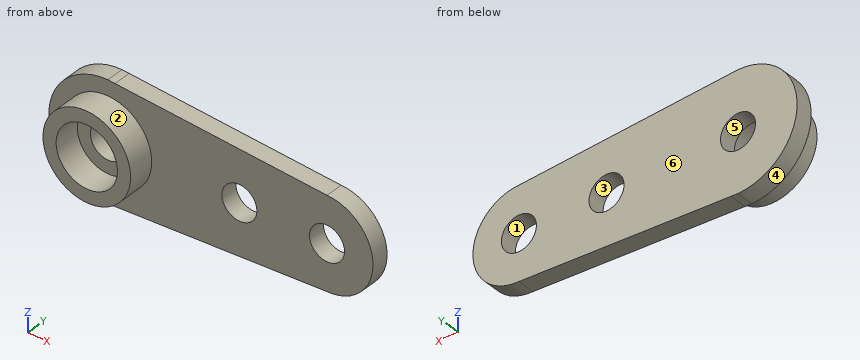
```python
from build123d import *

# Parameters (mm, degrees)
SKETCH_2_R      = 1
EXTRUDE_1_DEPTH = 1
SKETCH_3_R      = 2.5
SKETCH_3_R_2    = 1.75
EXTRUDE_2_DEPTH = 1.5


with BuildPart() as part:
    # 草图2 → 凸台-拉伸1 (new body)
    with BuildSketch(Plane(origin=(0, 0, 0), x_dir=(1, 0, 0), z_dir=(0, 1, 0))):
        with BuildLine():
            Line((0.40354723, 3.350787166), (0, 3.375))
            ThreePointArc((0, 3.375), (-3.375, 0), (0, -3.375))
            Line((0, -3.375), (0.40354723, -3.350787166))
            Line((0.40354723, -3.350787166), (12.5, -2.625))
            ThreePointArc((12.5, -2.625), (15.125, 0), (12.5, 2.625))
            Line((12.5, 2.625), (0.40354723, 3.350787166))
        make_face()
        with Locations(Location((0, 0, 0), (0, 0, 270))):
            Circle(SKETCH_2_R, mode=Mode.SUBTRACT)
        with Locations(Location((7.5, 0, 0), (0, 0, 270))):
            Circle(SKETCH_2_R, mode=Mode.SUBTRACT)
        with Locations(Location((12.5, 0, 0), (0, 0, 270))):
            Circle(SKETCH_2_R, mode=Mode.SUBTRACT)
    extrude(amount=EXTRUDE_1_DEPTH)

    # 草图3 → 凸台-拉伸2 (add)
    with BuildSketch(Plane(origin=(0, 0, 0), x_dir=(1, 0, 0), z_dir=(0, 1, 0))):
        with Locations(Location((0, 0, 0), (0, 0, 270))):
            Circle(SKETCH_3_R)
        with Locations(Location((0, 0, 0), (0, 0, 270))):
            Circle(SKETCH_3_R_2, mode=Mode.SUBTRACT)
    extrude(amount=-EXTRUDE_2_DEPTH)


solid = part.part
```
CAD build for the part. Positions are in the model's coordinates, mm. Face numbers are marked on the shaded views. A direction names the side the tool comes from. Coordinates: 2 decimals unless noted, no trailing zeros. Write each loop counter-clockwise with the first axis right and the second up, starting at its lowest first coordinate (ties: lowest second). Pieces come first, ordered by that corner, then holes.
(1) Drill centre lines: probe 1 along X at (y, z) = (0.7, 0) (3 decimals); probe 2 along Y at (x, z) = (10, 1.5); probe 3 along X at (y, z) = (-1.2, -1). Where is each one in solid material? Low to high.
(2) Flat gauge pin, fed straight in: pin 1 (4 mm diameter, centred on x = 5.5, z = -2, fed in from -Y). Where does the tip first touch, or does it go through?
(3) Cut at A-A, the plane z = 0. List the corners of the cut face in (x, y) (3 decimals).
(4) 3-axis set-ups, long thin cutter, end or side, ignore diameter. For the marked faces 1 and 2: which of +Z, -Z, +X, -X, +Y, -Y reach the whole face in a straight line?
(5) Cut at C-C, the plane x = 6.75. List the corners of the cut face in (y, z), and give its area (3 significant figures).
(6) Two-plate mould, pull along X, no slides. Class the marked faces 3, 4, 5 and 6: +X half, -X half, draft (parallel to the pull), parting line (faces both ways), or undercut.
(7) Cut at B-B, the plane y = 0.2. List the corners of the cut face in (x, z) (3 decimals).
(8) Cut at D-D, the plane x = 9.75. List the corners of the cut face in (y, z).
Geometry says:
1. probe 1: x = -3.375 to -1, 1 to 6.5, 8.5 to 11.5, 13.5 to 15.125
1. probe 2: y = 0 to 1
1. probe 3: x = -2.29 to -1.44, 1.44 to 2.29
2. pin 1: stops at y = 0
3. outline: (-3.375, 0) - (-2.5, 0) - (-2.5, -1.5) - (-1.75, -1.5) - (-1.75, 0) - (-1, 0) - (-1, 1) - (-3.375, 1) - close; (1, 0) - (1.75, 0) - (1.75, -1.5) - (2.5, -1.5) - (2.5, 0) - (6.5, 0) - (6.5, 1) - (1, 1) - close; (8.5, 0) - (11.5, 0) - (11.5, 1) - (8.5, 1) - close; (13.5, 0) - (15.125, 0) - (15.125, 1) - (13.5, 1) - close
4. face 1: +Y, -Y
4. face 2: -Y
5. outline: (0, -2.97) - (1, -2.97) - (1, -0.66) - (0, -0.66) - close; (0, 0.66) - (1, 0.66) - (1, 2.97) - (0, 2.97) - close
5. area: 4.62 mm2
6. face 3: undercut
6. face 4: -X half
6. face 5: undercut
6. face 6: draft
7. outline: (0, -3.375) - (12.5, -2.625) arc R2.625 ccw to (12.5, 2.625) - (0, 3.375) arc R3.375 ccw to start; hole circle Ø2 at (0, 0); hole circle Ø2 at (7.5, 0); hole circle Ø2 at (12.5, 0)
8. outline: (0, -2.79) - (1, -2.79) - (1, 2.79) - (0, 2.79) - close
